Source: CAD feature listing. Evaluate the final solid. Frame: model axes, mm. Face numbers are marked on the shaded views. A direction names the side the tool comes from. Give positions to 0.01 mm unless a question says otherwise; leave off trailing zeros. Loops run counter-clockwise (first coordinate to the right, second up) from the corner with the lowest first, then second, coordinate; pieces in that order, holes last. Notation, with made-up numbers: M 73,4 L 97,4 A25 cw 97,20 Z; hole C 81,-39.5 d11. An arc over 180 degrees is marked long. Answer in a Markdown table with one row per item.
```python
from build123d import *

# Parameters (mm, degrees)
SKETCH1_R           = 15
BOSS_EXTRUDE1_DEPTH = 44
SKETCH2_W           = 29.978808487
SKETCH2_H           = 7
CUT_EXTRUDE1_DEPTH  = 36
BOSS_EXTRUDE2_START = 30
SKETCH4_R           = 15
BOSS_EXTRUDE2_DEPTH = 30
SKETCH5_R           = 25
BOSS_EXTRUDE3_DEPTH = 10
SKETCH6_R           = 2.5
CUT_EXTRUDE2_DEPTH  = 92.137259121


with BuildPart() as part:
    # Sketch1 → Boss-Extrude1 (new body)
    with BuildSketch(Plane(origin=(0, 0, 0), x_dir=(1, 0, 0), z_dir=(0, 1, 0))):
        with Locations(Location((0, 0, 0), (0, 0, 270))):
            Circle(SKETCH1_R)
    extrude(amount=BOSS_EXTRUDE1_DEPTH)

    # Sketch2 → Cut-Extrude1 (cut)
    with BuildSketch(Plane(origin=(0, 44, 0), x_dir=(1, 0, 0), z_dir=(0, 1, 0))):
        with Locations((0.010595757, -3.5)):
            Rectangle(SKETCH2_W, SKETCH2_H)
    extrude(amount=-CUT_EXTRUDE1_DEPTH, mode=Mode.SUBTRACT)

    # Sketch4 → Boss-Extrude2 (add)
    with BuildSketch(Plane.XZ.offset(BOSS_EXTRUDE2_START)):
        with Locations(Location((0, 0, 0), (0, 0, 270))):
            Circle(SKETCH4_R)
    extrude(amount=-BOSS_EXTRUDE2_DEPTH)

    # Sketch5 → Boss-Extrude3 (add)
    with BuildSketch(Plane.XZ.offset(30)):
        with Locations(Location((0, 0, 0), (0, 0, 270))):
            Circle(SKETCH5_R)
    extrude(amount=BOSS_EXTRUDE3_DEPTH)

    # Sketch6 → Cut-Extrude2 (cut, through all)
    with BuildSketch(Plane.XZ.offset(40)):
        with BuildLine():
            ThreePointArc((0, 22.5), (-2.5, 20), (0, 17.5))
            Line((0, 17.5), (0, 22.5))
        make_face()
        with BuildLine():
            Line((0, 22.5), (0, 17.5))
            ThreePointArc((0, 17.5), (1.767766953, 18.232233047), (2.5, 20))
            ThreePointArc((2.5, 20), (1.767766953, 21.767766953), (0, 22.5))
        make_face()
        with Locations(Location((20, 0, 0), (0, 0, 270))):
            Circle(SKETCH6_R)
        with Locations(Location((0, -20, 0), (0, 0, 270))):
            Circle(SKETCH6_R)
        with Locations(Location((-20, 0, 0), (0, 0, 270))):
            Circle(SKETCH6_R)
    extrude(amount=-CUT_EXTRUDE2_DEPTH, mode=Mode.SUBTRACT)


solid = part.part
```
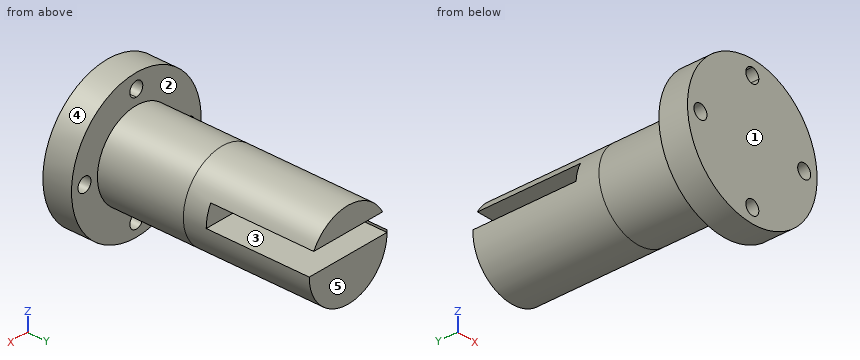
Q1. Ray query, probe 1 along X at (y, z) = (-33.25, 0); probe 2 along X at (y, z) = (-35, -20); probe 3 along Y at (x, z) = (-8.5, -13.5). Return the intervals inside material, ascending. Write a range as from..to.
Values follow:
| item | result |
|---|---|
| probe 1 | -25..-22.5, -17.5..17.5, 22.5..25 |
| probe 2 | -15..-2.5, 2.5..15 |
| probe 3 | -40..-30 |
Q2. Mould query, pull axis Z, two halves, no side actions, for the marked faces 3, 4 and 5. Classes: +Z half, -Z half, draft (parallel to the pull), parting line (faces both ways), or undercut.
Values follow:
| item | result |
|---|---|
| face 3 | undercut |
| face 4 | parting line |
| face 5 | draft |
Q3. Section query B-B (z = -20). Output: boundary loops of the cut face in (x, y).
Values follow:
| item | result |
|---|---|
| outline | M -15,-40 L -2.5,-40 L -2.5,-30 L -15,-30 Z; M 2.5,-40 L 15,-40 L 15,-30 L 2.5,-30 Z |
Q4. Contact query for flat-ended pins moving along their axis: pin 1 Ø8 at (x, z) = (20, 0) entering from -Y; pin 2 Ø6.5 at (x, z) = (0, -20) entering from +Y; pin 3 Ø9 at (x, y) = (-1, 32) entering from +Z; pin 4 Ø3 at (x, y) = (-13, -26) entering from -Z. Output: stop coordinate, or through.
Values follow:
| item | result |
|---|---|
| pin 1 | y = -40 |
| pin 2 | y = -30 |
| pin 3 | z = 15 |
| pin 4 | z = -9.63 |
Q5. Section query C-C (y = 17). Output: boundary loops of the cut face in (x, z).
Values follow:
| item | result |
|---|---|
| outline | M -14.98,0 L -14.98,0.8 A15 ccw long 15,0 Z; M -13.27,7 L 13.27,7 A15 ccw Z |
Q6. Reachability of the marked faces 1 and 2 from +Z, -Z, +X, -X, +Y, -Y: full face, straight path, thin tool, end or side. Return the list, or none.
Values follow:
| item | result |
|---|---|
| face 1 | +Z, -Z, +X, -X, -Y |
| face 2 | +Y |
Q7. Section query D-D (x = 12). Output: boundary loops of the cut face in (y, z), plus the area to 3 significant figures.
Values follow:
| item | result |
|---|---|
| outline | M -40,-21.93 L -30,-21.93 L -30,-9 L 44,-9 L 44,0 L 8,0 L 8,7 L 44,7 L 44,9 L -30,9 L -30,21.93 L -40,21.93 Z |
| area | 1,520 mm^2 |
Q8. Section query A-A (x = -20). Output: boundary loops of the cut face in (y, z), plus the area to 3 significant figures.
Values follow:
| item | result |
|---|---|
| outline | M -40,-15 L -30,-15 L -30,-2.5 L -40,-2.5 Z; M -40,2.5 L -30,2.5 L -30,15 L -40,15 Z |
| area | 250 mm^2 |
